Verification items for the finished model (mm, model axes). A direction names the side the tool comes from. Round coordinates to 2 decimals unless told otherwise and drop trailing zeros. Order: outer loops, then holes, each group sorted by start corner. A loop starts at its lowest first (then second) coordinate and runs counter-clockwise, first axis right, second up. Notation, with made-up numbers: M 9.5,17.5 L 13.5,17.5 A34 cw 13.5,54.5 Z; hole C 41,23.25 d11. An arc over 180 degrees is marked long. Use one line per item in the form item = value. Start each with the question number.
Item 1: Thickness scan on probe 1 along Z at (x, y) = (-70, 35.5); probe 2 along X at (y, z) = (24.5, 17.5); probe 3 along X at (y, z) = (40.5, 53.5). Record the ranges inside material, lowest first. Write a range as [from, to].
Item 2: Release check for a two-part mould opening along Y. For faces 1 (the flat face through (-14, 0, 10)), 2 (the flat face through (-14, 2, 10)), 3 (the flat face through (-14, 26, 64.211)), 4 (the flat face through (-94, 9.6, -1)) record: +Y half, -Y half, draft (parallel to the pull), parting line (faces both ways), or undercut.
Item 3: Tool access check on faces 5 (the flat face through (-87, 50, -34)), 6 (the flat face through (70.81, 26, 11)), 7 (the flat face through (-94, 15, -6.669)). Record the directions out of +Z, -Z, +X, -X, +Y, -Y that give a thin tool (end or side, any length) a straight path to the whole face; none if there is none.
Item 4: Cross-section at C-C on y = 44.8. Count the separate pieces of the cut face and the enclosed holes in it, then the cut area to 3 significant figures.
Item 5: Cross-section at A-A on z = -22. Enter the section's corners in (x, y), then the cut area to 3 significant figures.
Item 6: Cross-section at B-B on y = 24. Enter the section's corners in (x, z), then the cut area to 3 significant figures.
Item 7: Go/stop test with flat-tipped pins: pin 1 Ø7.5 at (x, y) = (13.81, 44.8) entering from +Z; pin 2 Ø4 at (x, z) = (-87, 54) entering from +Y; pin 3 Ø11.5 at (y, z) = (42.8, -7.11) entering from +X. Record where each tip stops, or that it passes through.
from build123d import *

# Parameters (mm, degrees)
SKETCH1_W                   = 167
SKETCH1_H                   = 107
BOSS_EXTRUDE1_DEPTH         = 52.8
SKETCH2_W                   = 157.8
SKETCH2_H                   = 97.5
CUT_EXTRUDE1_DEPTH          = 50.8
SKETCH3_R                   = 4.8
CUT_EXTRUDE2_DEPTH          = 108
LPATTERN1_COUNT             = 8
LPATTERN1_PITCH             = 18
SKETCH4_R                   = 6.35
CUT_EXTRUDE3_DEPTH          = 4.55
LPATTERN2_COUNT             = 2
LPATTERN2_PITCH             = 35.66
CUT_EXTRUDE4_REACH          = 169
SKETCH5_W                   = 11.94
SKETCH5_H                   = 10.8
BOSS_EXTRUDE5_DEPTH         = 48
M3_TAPPED_HOLE1_D           = 2.5
M3_TAPPED_HOLE1_CSINK_D     = 3.05
M3_TAPPED_HOLE1_CSINK_ANGLE = 90


with BuildPart() as part:
    # Sketch1 → Boss-Extrude1 (new body)
    with BuildSketch(Plane(origin=(0, 0, 0), x_dir=(1, 0, 0), z_dir=(0, 1, 0))):
        with Locations((-12.690388251, -10.711139896)):
            Rectangle(SKETCH1_W, SKETCH1_H)
    extrude(amount=BOSS_EXTRUDE1_DEPTH)

    # Sketch2 → Cut-Extrude1 (cut)
    with BuildSketch(Plane(origin=(0, 52.8, 0), x_dir=(1, 0, 0), z_dir=(0, 1, 0))):
        with Locations((-12.640388251, -10.711139896)):
            Rectangle(SKETCH2_W, SKETCH2_H)
    extrude(amount=-CUT_EXTRUDE1_DEPTH, mode=Mode.SUBTRACT)

    # Sketch3 → Cut-Extrude2 (cut, through all)
    with BuildSketch(Plane.XY.offset(64.211139896)):
        with Locations((-76.190388251, 44.8)):
            Circle(SKETCH3_R)
    cut_extrude2 = extrude(amount=-CUT_EXTRUDE2_DEPTH, mode=Mode.SUBTRACT)

    # LPattern1: Cut-Extrude2 ×8
    with Locations(*[(i * LPATTERN1_PITCH, 0, 0) for i in range(1, LPATTERN1_COUNT)]):
        add(cut_extrude2, mode=Mode.SUBTRACT)

    # Sketch4 → Cut-Extrude3 (cut)
    with BuildSketch(Plane(origin=(70.809611749, 0, 0), x_dir=(0, 0, -1), z_dir=(1, 0, 0))):
        with Locations((-28.551139896, 42.8)):
            Circle(SKETCH4_R)
    cut_extrude3 = extrude(amount=-CUT_EXTRUDE3_DEPTH, mode=Mode.SUBTRACT)

    # LPattern2: Cut-Extrude3 ×2
    with Locations(*[(0, 0, -i * LPATTERN2_PITCH) for i in range(1, LPATTERN2_COUNT)]):
        add(cut_extrude3, mode=Mode.SUBTRACT)

    # Sketch5 → Cut-Extrude4 (cut, up to next)
    with BuildSketch(Plane.ZY.offset(96.190388251), mode=Mode.PRIVATE) as cut_extrude4_sk1:
        with Locations((-0.698860104, 15)):
            Rectangle(SKETCH5_W, SKETCH5_H)
    cut_extrude4_tool1 = extrude(cut_extrude4_sk1.sketch, amount=-CUT_EXTRUDE4_REACH, mode=Mode.PRIVATE) & part.part
    add(cut_extrude4_tool1.solids().sort_by_distance((-96.190388, 15, -0.69886))[0], mode=Mode.SUBTRACT)

    # Sketch6 → Boss-Extrude5 (add)
    with BuildSketch(Plane(origin=(0, 2, 0), x_dir=(1, 0, 0), z_dir=(0, 1, 0))):
        with BuildLine():
            Line((66.259611749, 34.038860104), (66.259611749, 38.038860104))
            Line((66.259611749, 38.038860104), (62.259611749, 38.038860104))
            ThreePointArc((62.259611749, 38.038860104), (59.431184624, 31.210432979), (66.259611749, 34.038860104))
        make_face()
        with BuildLine():
            Line((66.259611749, -59.461139896), (62.259611749, -59.461139896))
            ThreePointArc((62.259611749, -59.461139896), (59.431184624, -52.632712772), (66.259611749, -55.461139896))
            Line((66.259611749, -55.461139896), (66.259611749, -59.461139896))
        make_face()
        with BuildLine():
            Line((-91.540388251, 38.038860104), (-87.540388251, 38.038860104))
            ThreePointArc((-87.540388251, 38.038860104), (-84.711961126, 31.210432979), (-91.540388251, 34.038860104))
            Line((-91.540388251, 34.038860104), (-91.540388251, 38.038860104))
        make_face()
        with BuildLine():
            Line((-91.540388251, -55.461139896), (-91.540388251, -59.461139896))
            Line((-91.540388251, -59.461139896), (-87.540388251, -59.461139896))
            ThreePointArc((-87.540388251, -59.461139896), (-84.711961126, -52.632712772), (-91.540388251, -55.461139896))
        make_face()
    extrude(amount=BOSS_EXTRUDE5_DEPTH)

    # M3 Tapped Hole1 (through all)
    with Locations(Plane(origin=(-49.02040068, 2, -140.944816831), x_dir=(1, 0, 0), z_dir=(0, 1, 0))):
        with Locations((56.769595429, -175.881156727), (25.768895429, -171.002663961), (-25.856604571, -175.881156727), (-25.856604571, -127.544956727), (49.276595429, -127.544956727), (25.768895429, -142.986463961)):
            CounterSinkHole(M3_TAPPED_HOLE1_D / 2, M3_TAPPED_HOLE1_CSINK_D / 2, counter_sink_angle=M3_TAPPED_HOLE1_CSINK_ANGLE)


solid = part.part
Output values:
q1.probe_1 = [-42.79, -38.04], [59.46, 64.21]
q1.probe_2 = [-96.19, -91.54], [66.26, 70.81]
q1.probe_3 = [-96.19, -91.54], [-91.03, -84.05], [58.77, 65.75], [66.26, 70.81]
q2.face_1 = -Y half
q2.face_2 = +Y half
q2.face_3 = draft
q2.face_4 = undercut
q3.face_5 = +Y
q3.face_6 = +Z, -Z, +X, +Y, -Y
q3.face_7 = -X
q4.separate_pieces = 18
q4.enclosed_holes = 0
q4.area = 1,860 mm2
q5.outline = M -96.19,0 L 70.81,0 L 70.81,52.8 L 66.26,52.8 L 66.26,2 L -91.54,2 L -91.54,52.8 L -96.19,52.8 Z
q5.area = 801 mm2
q6.outline = M -96.19,-42.79 L 70.81,-42.79 L 70.81,64.21 L -96.19,64.21 Z; hole M -91.54,-34.04 A4 cw long -87.54,-38.04 L 62.26,-38.04 A4 cw long 66.26,-34.04 L 66.26,55.46 A4 cw long 62.26,59.46 L -87.54,59.46 A4 cw long -91.54,55.46 Z
q6.area = 2,700 mm2
q7.pin_1 = through
q7.pin_2 = 50
q7.pin_3 = -91.54
